Verification items for the finished model (mm, model axes). A direction names the side the tool comes from. Give positions to 0.01 mm unless a question says otherwise; leave off trailing zeros. Loops run counter-clockwise (first coordinate to the right, second up) from the corner with the lowest first, then second, coordinate; pieces in that order, holes last. Notation, with made-up numbers: (5, 42.5) - (29, 42.5) arc R24 ccw to (29, 53.5) - close; hole circle Ø3 at (-14, 64). An arc over 180 degrees is marked (long way). Use one line per item in the form item = value.
```python
from build123d import *

# Parameters (mm, degrees)
ESBO_O2_R                = 15
RESSALTO_EXTRUS_O3_DEPTH = 15
ESBO_O1_R                = 2.4
CORTE_EXTRUS_O4_DEPTH    = 15
RESSALTO_EXTRUS_O4_DEPTH = 9
ESBO_O5_R                = 4.5
RESSALTO_EXTRUS_O5_DEPTH = 9
CORTE_EXTRUS_O7_DEPTH    = 7.5
FILETE3_R                = 0.5


with BuildPart() as part:
    # Esboço2 → Ressalto-extrusão3 (new body)
    with BuildSketch(Plane(origin=(0, 0, 0), x_dir=(1, 0, 0), z_dir=(0, 1, 0))):
        with Locations(Location((0, 0, 0), (0, 0, 270))):
            Circle(ESBO_O2_R)
    extrude(amount=RESSALTO_EXTRUS_O3_DEPTH)

    # Esboço1 → Corte-extrusão4 (cut)
    with BuildSketch(Plane(origin=(0, 0, 0), x_dir=(1, 0, 0), z_dir=(0, 1, 0))):
        with Locations(Location((-6.59, 3.46, 0), (0, 0, 270))):
            Circle(ESBO_O1_R)
        with Locations(Location((6.59, 3.46, 0), (0, 0, 270))):
            Circle(ESBO_O1_R)
        with Locations(Location((6.59, -3.46, 0), (0, 0, 90))):
            Circle(ESBO_O1_R)
        with Locations(Location((0, 8, 0), (0, 0, 270))):
            Circle(ESBO_O1_R)
        with Locations(Location((0, -8, 0), (0, 0, 90))):
            Circle(ESBO_O1_R)
        with Locations(Location((-6.59, -3.46, 0), (0, 0, 90))):
            Circle(ESBO_O1_R)
    extrude(amount=CORTE_EXTRUS_O4_DEPTH, mode=Mode.SUBTRACT)

    # Esboço3 → Ressalto-extrusão4 (add)
    with BuildSketch(Plane(origin=(0, 15, 0), x_dir=(1, 0, 0), z_dir=(0, 1, 0))):
        with BuildLine():
            Line((0.8, -0.8), (2.2627417, -0.8))
            ThreePointArc((2.2627417, -0.8), (2.4, 0), (2.2627417, 0.8))
            Line((2.2627417, 0.8), (0.8, 0.8))
            Line((0.8, 0.8), (0.8, 2.2627417))
            ThreePointArc((0.8, 2.2627417), (0, 2.4), (-0.8, 2.2627417))
            Line((-0.8, 2.2627417), (-0.8, 0.8))
            Line((-0.8, 0.8), (-2.2627417, 0.8))
            ThreePointArc((-2.2627417, 0.8), (-2.4, 0), (-2.2627417, -0.8))
            Line((-2.2627417, -0.8), (-0.8, -0.8))
            Line((-0.8, -0.8), (-0.8, -2.2627417))
            ThreePointArc((-0.8, -2.2627417), (0, -2.4), (0.8, -2.2627417))
            Line((0.8, -2.2627417), (0.8, -0.8))
        make_face()
    extrude(amount=RESSALTO_EXTRUS_O4_DEPTH)

    # Esboço5 → Ressalto-extrusão5 (add)
    with BuildSketch(Plane.XZ):
        with Locations(Location((0, 0, 0), (0, 0, 90))):
            Circle(ESBO_O5_R)
    extrude(amount=RESSALTO_EXTRUS_O5_DEPTH)

    # Esboço6 → Corte-extrusão7 (cut)
    with BuildSketch(Plane.XZ.offset(9)):
        with BuildLine():
            Line((1.878473588, -0.68653986), (0.915964349, 1.777922752))
            ThreePointArc((0.915964349, 1.777922752), (-1.862958624, -0.727588595), (1.878473588, -0.68653986))
        make_face()
    extrude(amount=-CORTE_EXTRUS_O7_DEPTH, mode=Mode.SUBTRACT)

    # Filete3
    filete3_edges = [part.edges().sort_by_distance(p)[0] for p in [
        (0, 0, -15),
        (1.53137085, 15, 0.8),
        (2.4, 15, 0),
        (0.8, 15, -1.53137085),
        (0, 15, -2.4),
        (-1.53137085, 15, -0.8),
        (-2.4, 15, 0),
        (0, 15, -15),
        (-0.8, 15, 1.53137085),
        (0, 15, 2.4),
        (0.8, 15, 1.53137085),
        (-1.53137085, 15, 0.8),
        (-0.8, 15, -1.53137085),
        (1.53137085, 15, -0.8),
        (0, 0, -4.5),
        (0, -9, -4.5),
    ]]
    fillet(filete3_edges, radius=FILETE3_R)


solid = part.part
```
1. Scan lines: probe 1 along Z at (x, y) = (0.75, 12); probe 2 along X at (y, z) = (10.25, 3.46); probe 3 along X at (y, z) = (10, -3). Record each from-to range of solid material in increasing order.
Result set:
probe_1 = -14.98 to -10.28, -5.72 to 5.72, 10.28 to 14.98
probe_2 = -14.6 to -8.99, -4.19 to 4.19, 8.99 to 14.6
probe_3 = -14.7 to -8.95, -4.23 to 4.23, 8.95 to 14.7
2. Draft check along Z on faces 1 (the cylindrical face through (0, 19.7, 2.4)), 2 (the flat face through (-0.8, 20, -2)), 3 (the cylindrical face through (-0.106, 7.395, 10.398)). Enter one of: released by +Z, released by -Z, zero draft, split by the parting line, or undercut.
Result set:
face_1 = released by +Z
face_2 = zero draft
face_3 = undercut
3. Section check D-D, the plane y = 22. Record the cut outline in (x, z).
Result set:
outline = (-2.26, -0.8) - (-0.8, -0.8) - (-0.8, -2.26) arc R2.4 ccw to (0.8, -2.26) - (0.8, -0.8) - (2.26, -0.8) arc R2.4 ccw to (2.26, 0.8) - (0.8, 0.8) - (0.8, 2.26) arc R2.4 ccw to (-0.8, 2.26) - (-0.8, 0.8) - (-2.26, 0.8) arc R2.4 ccw to start
4. Section check B-B, the plane y = 13. Record the cut outline in (x, z), then the cut area to 3 significant figures.
Result set:
outline = circle Ø30 at (0, 0); hole circle Ø4.8 at (-6.59, -3.46); hole circle Ø4.8 at (-6.59, 3.46); hole circle Ø4.8 at (0, -8); hole circle Ø4.8 at (0, 8); hole circle Ø4.8 at (6.59, -3.46); hole circle Ø4.8 at (6.59, 3.46)
area = 598 mm²
5. Section check C-C, the plane z = 0. Record the cut outline in (x, y), then the cut area to 3 significant figures.
Result set:
outline = (-15, 0.5) arc R0.5 ccw to (-14.5, 0) - (-5, 0) arc R0.5 cw to (-4.5, -0.5) - (-4.5, -8.5) arc R0.5 ccw to (-4, -9) - (-2, -9) - (-2, -1.5) - (1.61, -1.5) - (1.61, -9) - (4, -9) arc R0.5 ccw to (4.5, -8.5) - (4.5, -0.5) arc R0.5 cw to (5, 0) - (14.5, 0) arc R0.5 ccw to (15, 0.5) - (15, 14.5) arc R0.5 ccw to (14.5, 15) - (2.9, 15) arc R0.5 cw to (2.4, 15.5) - (2.4, 24) - (-2.4, 24) - (-2.4, 15.5) arc R0.5 cw to (-2.9, 15) - (-14.5, 15) arc R0.5 ccw to (-15, 14.5) - close
area = 547 mm²
6. Depth check by flat-ended pin: pin 1 Ø1.6 at (y, z) = (18.5, -1.5) entering from -X; pin 2 Ø4.5 at (x, z) = (-6.59, -3.46) entering from +Y; pin 3 Ø5.5 at (x, z) = (6.59, 3.46) entering from +Y; pin 4 Ø8 at (x, y) = (5.5, -1.5) entering from +Z. Enter the tip coordinate at first touch or a pass-through.
Result set:
pin_1 = -2.3
pin_2 = through
pin_3 = 15
pin_4 = 14.86
7. Tool access check on faces 4 (the cylindrical face through (0, 19.7, -2.4)), 5 (the flat face through (2, 20, -0.8)), 6 (the flat face through (2, 20, 0.8)). Record the directions out of +Z, -Z, +X, -X, +Y, -Y that give a thin tool (end or side, any length) a straight path to the whole face; none if there is none.
Result set:
face_4 = -Z, +Y
face_5 = -Z, +X, +Y
face_6 = +Z, +X, +Y
8. Section check A-A, the plane x = 0. State how many separate pieces and enclosed holes the cut face has, then the cut area to 3 significant figures.
Result set:
separate_pieces = 3
enclosed_holes = 0
area = 400 mm²
